Here's how the part is built. I have some questions about the finished solid (model axes, mm). A direction names the side the tool comes from. Round coordinates to 2 decimals unless told otherwise and drop trailing zeros. Loops run counter-clockwise (first coordinate to the right, second up) from the corner with the lowest first, then second, coordinate; pieces in that order, holes last. Notation, with made-up numbers: (28.5, 13) - (49.5, 13) arc R18 ccw to (49.5, 40) - close; hole circle Ø5 at (-36, 57.5). An arc over 180 degrees is marked (long way). Return JSON: item names as keys, results as strings. Group by question number.
```python
from build123d import *

# Parameters (mm, degrees)
F0_W     = 75
F0_H     = 25
F1_DEPTH = 150


with BuildPart() as f1:
    # F0 (on Front) → F1 (new body)
    with BuildSketch(Plane.XZ):
        with Locations((-37.5, 62.5)):
            Rectangle(F0_W, F0_H)
        Polygon((50, 0), (0, 75), (0, 50), (25, 0), align=None)
        Polygon((-75, 50), (-75, 75), (-125, 0), (-100, 0), align=None)
        Polygon((0, -75), (50, 0), (25, 0), (0, -50), align=None)
        Polygon((-100, 0), (-125, 0), (-75, -75), (-75, -50), align=None)
        with Locations((-37.5, -62.5)):
            Rectangle(F0_W, F0_H)
    extrude(amount=F1_DEPTH)


solid = f1.part
```
Q1. Will these pins go through, and if not, where does the flat tip stop? pin 1 Ø4 at (y, z) = (-36, 10.5) entering from -X; pin 2 Ø5 at (x, y) = (-95, -22.5) entering from +Z; pin 3 Ø1.5 at (y, z) = (-62.5, 19) entering from +X.
Q2. If we mould it in two halves opening along Z, with no side actions, what happens to faces 3 (the flat face through (-99.65, -73.95, 38.025)), 4 (the flat face through (-38, -74, 50)), 5 (the flat face through (-38, -74, -50)), 6 (the flat face through (-100.35, -73.95, -36.975))? For each: +Z half, -Z half, draft (parallel to the pull), parting line (faces both ways), or undercut.
Q3. Imagine slicing it at A-A, the plane z = 31.5. List the corners of the cut face in (x, y) for me.
Q4. Please list where these lines run through material, in increasing order: line 1 (Z direction, x = -51, y = -87); line 2 (Z direction, x = 9, y = -45.5); line 3 (X direction, y = -32, z = 22).
Q5. Imagine slicing it at B-B, the plane x = -94.5. List the corners of the cut face in (y, z) for me.
Q6. Imagine slicing it at C-C, the plane y = -77. List the corners of the cut face in (x, z) for me, and give its area (3 significant figures).
Q7. Imagine slicing it at D-D, the plane x = 29. List the corners of the cut face in (y, z) for me.
Q8. For faces 1 (the flat face through (-38, -74, 75)), 2 (the flat face through (12.325, -73.95, 25.35)), which set-ups out of +Z, -Z, +X, -X, +Y, -Y let a thin tool reach every point of the face, with its end or its side?
Output values:
{
 "1": {"pin 1": "stops at x = -119.33", "pin 2": "stops at z = 48.75", "pin 3": "stops at x = 37.83"},
 "2": {"face 3": "+Z half", "face 4": "undercut", "face 5": "undercut", "face 6": "-Z half"},
 "3": {"outline": "(-104, -150) - (-84.25, -150) - (-84.25, 0) - (-104, 0) - close; (9.25, -150) - (29, -150) - (29, 0) - (9.25, 0) - close"},
 "4": {"line 1": "z = -75 to -50, 50 to 75", "line 2": "z = -61.5 to -32, 32 to 61.5", "line 3": "x = -110.33 to -89, 14 to 35.33"},
 "5": {"outline": "(-150, -45.75) - (0, -45.75) - (0, -11) - (-150, -11) - close; (-150, 11) - (0, 11) - (0, 45.75) - (-150, 45.75) - close"},
 "6": {"outline": "(-125, 0) - (-75, -75) - (0, -75) - (50, 0) - (0, 75) - (-75, 75) - close; hole (-100, 0) - (-75, -50) - (0, -50) - (25, 0) - (0, 50) - (-75, 50) - close", "area": "8,750 mm^2"},
 "7": {"outline": "(-150, -31.5) - (0, -31.5) - (0, 31.5) - (-150, 31.5) - close"},
 "8": {"face 1": "+Z, +X, -X, +Y, -Y", "face 2": "+Y, -Y"}
}
